Solid Edge part; units mm, degrees
sketch "Sketch1" plane through (0, 0, 0) normal (0, 0, 1) x (1, 0, 0)
  circle A0 centre (-27.6601, 27.4589) radius 25
extrude "Protrusion1" add sketch "Sketch1" along normal blind 50
fillet "Round_1" radius 5 1 edges at (-52.6601, 27.4589, 0)
fillet "Round_2" radius 3 1 edges at (-52.6601, 27.4589, 50)
sketch "Sketch2" plane through (-27.6601, 27.4589, 50) normal (0, 0, 1) x (0, -1, 0)
  circle A0 centre (0, 0) radius 10
extrude "ExtrudedProtrusion_2" add sketch "Sketch2" along normal blind 5
sketch "Sketch3" plane through (-27.6601, 27.4589, 0) normal (0, 0, -1) x (-1, 0, 0)
  circle A0 centre (0, 0) radius 10
extrude "ExtrudedProtrusion_3" add sketch "Sketch3" along normal blind 5
sketch "Sketch4" plane through (-27.6601, 27.4589, 55) normal (0, 0, 1) x (-1, 0, 0)
  circle A0 centre (0, 0) radius 3.556
extrude "ExtrudedProtrusion_4" add sketch "Sketch4" along normal blind 15.24
sketch "Sketch5" plane through (-27.6601, 27.4589, 0) normal (0, 0, -1) x (0, 1, 0)
  circle A0 centre (-19.0472, 0) radius 1.5
  circle A1 centre (19.0472, 0.1743) radius 1.5
extrude "ExtrudedProtrusion_6" add sketch "Sketch5" along normal blind 3.81
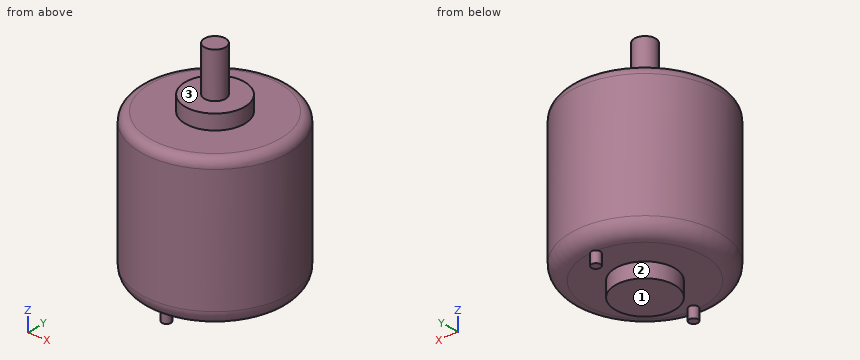
Geometry check sheet. Reference: the model listing, model coordinates, mm. Face numbers are marked on the shaded views. A direction names the side the tool comes from. Round coordinates to 2 decimals unless told otherwise and drop trailing zeros. Order: outer loops, then holes, each group sorted by start corner. A loop starts at its lowest first (then second) coordinate and runs counter-clockwise, first axis right, second up. Notation, with made-up numbers: M 17,20 L 46,20 A26 ccw 46,49 Z; hole C 44.25,84.25 d2. An arc over 180 degrees is marked long. Answer as CSV lines item,"result".
1) Tool access check on the marked faces 1, 2 and 3. Record the directions out of +Z, -Z, +X, -X, +Y, -Y that give a thin tool (end or side, any length) a straight path to the whole face; none if there is none.
Entries:
face 1,"-Z, +X, -X, +Y, -Y"
face 2,"-Z"
face 3,"+Z"
2) Thickness scan on probe 1 along Z at (x, y) = (-9, 22); probe 2 along Y at (x, z) = (-16, 4); probe 3 along Z at (x, y) = (-37, 27.5). Record the ranges inside material, lowest first. Write a range as [from, to].
Entries:
probe 1,"[0, 50]"
probe 2,"[5.46, 49.46]"
probe 3,"[-5, 55]"
3) Sectioned sample at B-B on z = 32. Record the cut outline in (x, y).
Entries:
outline,"C -27.66,27.46 d50"
4) Sectioned sample at A-A on z = 59. Record the cut outline in (x, y), and give its area (3 significant figures).
Entries:
outline,"C -27.66,27.46 d7.11"
area,"39.7 mm2"
5) Gauge pin test, flat ends, axial feed: pin 1 Ø3 at (x, y) = (-33, 9) entering from -Z; pin 2 Ø1 at (x, z) = (-34, 23.5) entering from +Y; pin 3 Ø1.5 at (x, z) = (-17.5, 38.5) entering from +Y. Record the tip position at first contact, or that the pin passes through.
Entries:
pin 1,"z = 0"
pin 2,"y = 51.77"
pin 3,"y = 50.62"
